Part model, mm, in its own coordinate system. A direction names the side the tool comes from. Round coordinates to 2 decimals unless told otherwise and drop trailing zeros. Loops run counter-clockwise (first coordinate to the right, second up) from the corner with the lowest first, then second, coordinate; pieces in that order, holes last. Notation, with made-up numbers: (-1, 14.25) -> (35, 14.25) arc R35 ccw to (35, 49.25) -> close; hole circle Ø4 at (-5.75, 25). An arc over 180 degrees is marked (long way). Use a Markdown table: item, result. Add a question column.
Item 1: Probe line 1 (Y direction, x = 39.5, z = 44.5); line 2 (Y direction, x = 105, z = 38.5); line 3 (X direction, y = -26.5, z = 35). List the from-to ranges inside material, lowest first. Write a range as [from, to].
Item 2: Which spindle directions (+Z, -Z, +X, -X, +Y, -Y) get a long thin tool onto all of the face, cutting with end or side? Do faces 4 (the face through (41, -4, 45)), 5 (the face through (103, -31, 37)), 6 (the face through (136, -33, 37)). Say none if no direction does.
Item 3: Flat gauge pins, fed straight in: pin 1 (15.5 mm diameter, centred on y = -16, z = 33.5, fed in from +X); pin 2 (3 mm diameter, centred on y = -14.5, z = 36.5, fed in from -X); pin 3 (20 mm diameter, centred on x = 27, z = 53, fed in from -Y). Where does each tip first touch, or does it go through?
Item 4: Cut at A-A, the plane x = 32. List the corners of the cut face in (y, z), plus the area to 3 significant figures.
Item 5: Cut at D-D, the plane y = -20. List the corners of the cut face in (x, z), plus the area to 3 significant figures.
Item 6: Cut at B-B, the plane z = 37.5. List the corners of the cut face in (x, y), plus the area to 3 significant figures.
Item 7: Cut at C-C, the plane z = 58. List the corners of the cut face in (x, y), plus the area to 3 significant figures.
Item 8: Two-plate mould, pull along Z, no slides. Class faces 1 (the face through (70, -15, 37)), 2 (the face through (69.7, -18.7, 0)), 3 (the face through (22.24, -1.97, 35.33)): pulls with the +Z half, pulls with the -Z half, needs draft (parallel to the pull), parting line crosses it, or undercut.
```python
from build123d import *

# Parameters (mm, degrees)
BOSS_EXTRUDE1_DEPTH = 75
SKETCH2_R           = 10
CUT_EXTRUDE1_DEPTH  = 160.204271299
CHAMFER1_SIZE       = 10
CHAMFER1_SIZE2      = 20
CHAMFER2_SIZE       = 20
CHAMFER2_SIZE2      = 10
CHAMFER3_SIZE       = 5
CHAMFER3_SIZE2      = 2.886751346


with BuildPart() as part:
    # Sketch1 → Boss-Extrude1 (new body)
    with BuildSketch(Plane.XY):
        Polygon((0, 0), (70, 0), (70, -31), (136, -31), (136, -35), (66, -35), (66, -4), (0, -4), align=None)
    extrude(amount=BOSS_EXTRUDE1_DEPTH)

    # Sketch2 → Cut-Extrude1 (cut, through all)
    with BuildSketch(Plane(origin=(0, 0, 0), x_dir=(1, 0, 0), z_dir=(0, 1, 0))):
        with Locations(Location((32, -37.5, 0), (0, 0, 270))):
            Circle(SKETCH2_R)
    extrude(amount=-CUT_EXTRUDE1_DEPTH, mode=Mode.SUBTRACT)

    # Chamfer1
    chamfer1_edges = [part.edges().sort_by_distance(p)[0] for p in [
        (0, -2, 75),
    ]]
    chamfer1_side = [part.faces().sort_by_distance(p)[0] for p in [
        (0, -2, 37.5),
    ]]
    chamfer(chamfer1_edges, length=CHAMFER1_SIZE, length2=CHAMFER1_SIZE2, reference=chamfer1_side[0])

    # Chamfer2
    chamfer2_edges = [part.edges().sort_by_distance(p)[0] for p in [
        (0, -2, 0),
    ]]
    chamfer2_side = [part.faces().sort_by_distance(p)[0] for p in [
        (68, -17.5, 0),
    ]]
    chamfer(chamfer2_edges, length=CHAMFER2_SIZE, length2=CHAMFER2_SIZE2, reference=chamfer2_side[0])

    # Chamfer3
    chamfer3_edges = [part.edges().sort_by_distance(p)[0] for p in [
        (0, 0, 37.5),
    ]]
    chamfer3_side = [part.faces().sort_by_distance(p)[0] for p in [
        (1.025914226, 0, 37.5),
    ]]
    chamfer(chamfer3_edges, length=CHAMFER3_SIZE, length2=CHAMFER3_SIZE2, reference=chamfer3_side[0])


solid = part.part
```
A:
| question | item | result |
|---|---|---|
| 1 | line 1 | y = [-4, 0] |
| 1 | line 2 | y = [-35, -31] |
| 1 | line 3 | x = [66, 70] |
| 2 | face 4 | +Z, -Z, -X, -Y |
| 2 | face 5 | +Z, -Z, +X, +Y |
| 2 | face 6 | +Z, -Z, +X, +Y, -Y |
| 3 | pin 1 | stops at x = 70 |
| 3 | pin 2 | stops at x = 66 |
| 3 | pin 3 | stops at y = -4 |
| 4 | outline | (-4, 0) -> (0, 0) -> (0, 27.5) -> (-4, 27.5) -> close; (-4, 47.5) -> (0, 47.5) -> (0, 75) -> (-4, 75) -> close |
| 4 | area | 220 mm^2 |
| 5 | outline | (66, 0) -> (70, 0) -> (70, 75) -> (66, 75) -> close |
| 5 | area | 300 mm^2 |
| 6 | outline | (0, -4) -> (22, -4) -> (22, 0) -> (5, 0) -> (0, -2.89) -> close; (42, -4) -> (66, -4) -> (66, -35) -> (136, -35) -> (136, -31) -> (70, -31) -> (70, 0) -> (42, 0) -> close |
| 6 | area | 581 mm^2 |
| 7 | outline | (0, -4) -> (66, -4) -> (66, -35) -> (136, -35) -> (136, -31) -> (70, -31) -> (70, 0) -> (5, 0) -> (0, -2.89) -> close |
| 7 | area | 661 mm^2 |
| 8 | face 1 | needs draft |
| 8 | face 2 | pulls with the -Z half |
| 8 | face 3 | undercut |
